Input: part model. Units: mm. Frame: model coordinates. A direction names the side the tool comes from. Give positions to 0.01 mm unless a question says otherwise; leave off trailing zeros. Write each loop counter-clockwise with the first axis right and the second up, starting at its lowest first coordinate (ties: lowest second). Pieces come first, ordered by that corner, then holes.
```python
from build123d import *

# Parameters (mm, degrees)
F1_DEPTH = 101
F2_W     = 28
F2_H     = 1
F3_DEPTH = 2


with BuildPart() as f1:
    # F0 (on Front) → F1 (new body)
    with BuildSketch(Plane.XZ):
        Polygon((19.7989898732, 1.4142135624), (0, 21.2132034356), (-0.4420594911, 18.826835802), (16.3847763109, 2), (-30.2015638745, 2), (-20.19282931, 38.5776056209), (-15.051559592, 33.4363359028), (-14.1421356237, 35.3553390593), (-21.2132034356, 42.4264068712), (-32.8223461799, 0), (-9.7140957444, 0), (21.2132034356, 0), align=None)
        Polygon((21.0717820794, 2.6870057685), (19.7989898732, 1.4142135624), (21.2132034356, 0), (23.9002092041, 2.6870057685), (21.0717820794, 5.5154328933), (19.657568517, 4.1012193309), align=None)
    extrude(amount=F1_DEPTH)

    # F2 (on face) → F3 (join)
    with BuildSketch(Plane(origin=(10.6066017178, 0, 10.6066017178), x_dir=(0.7071067812, 0, -0.7071067812), z_dir=(0.7071067812, 0, 0.7071067812))):
        with Locations((-1, -100.5)):
            Rectangle(F2_W, F2_H)
        with Locations((-1, -90.5)):
            Rectangle(F2_W, F2_H)
        with Locations((-1, -80.5)):
            Rectangle(F2_W, F2_H)
        with Locations((-1, -70.5)):
            Rectangle(F2_W, F2_H)
        with Locations((-1, -60.5)):
            Rectangle(F2_W, F2_H)
        with Locations((-1, -50.5)):
            Rectangle(F2_W, F2_H)
        with Locations((-1, -40.5)):
            Rectangle(F2_W, F2_H)
        with Locations((-1, -30.5)):
            Rectangle(F2_W, F2_H)
        with Locations((-1, -20.5)):
            Rectangle(F2_W, F2_H)
        with Locations((-1, -0.5)):
            Rectangle(F2_W, F2_H)
        with Locations((-1, -10.5)):
            Rectangle(F2_W, F2_H)
    extrude(amount=F3_DEPTH)


solid = f1.part
```
Q1. Section B-B, the plane x = -7. Return the cut outline in (y, z).
Q2. Section A-A, the plane y = -16.5. Return the cut outline in (x, z).
Q3. Section C-C, the plane z = 29.5. Return the cut outline in (x, y).
Q4. Pin query (flat end, axial travel): pin 1 (6 mm diameter, centred on y = -42.5, z = 26, fed in from +X); pin 2 (5 mm diameter, centred on y = -25, z = 31, fed in from +X); pin 3 (17 mm diameter, centred on x = 12.5, z = 11, fed in from +Y); pin 4 (6 mm diameter, centred on y = -36.5, z = 7, fed in from -X). Return the tip coordinate at first contact, or that it passes through.
Q5. Access query for faces 3 (the flat face through (-17.628, -49.793, 38.841)), 4 (the flat face through (-17.658, -49.793, 36.043)). Directions: +Z, -Z, +X, -X, +Y, -Y. A direction counts if a zero-diameter tool reaches every point of the face in a straight line with its end or side. Return the directions, or none.
Q6. Material intervals for line 1 along X through (y, z) = (-76, 3.5); line 2 along Z through (x, y) = (6, -39); line 3 along X through (y, z) = (-23.5, 4.5), sorted ascending.
Q7. Mould query, pull axis Y, two halves, no side actions, for faces 1 (the flat face through (10, -1, 12)), 2 (the flat face through (22.51, -49.79, 4.08)). Classes: +Y half, -Y half, draft (parallel to the pull), parting line (faces both ways), or undercut.
Solutions:
1. outline: (-101, 0) - (0, 0) - (0, 2) - (-101, 2) - close
2. outline: (-32.82, 0) - (21.21, 0) - (23.9, 2.69) - (21.07, 5.52) - (19.66, 4.1) - (21.07, 2.69) - (19.8, 1.41) - (0, 21.21) - (-0.44, 18.83) - (16.38, 2) - (-30.2, 2) - (-20.19, 38.58) - (-15.05, 33.44) - (-14.14, 35.36) - (-21.21, 42.43) - close
3. outline: (-24.75, -101) - (-22.68, -101) - (-22.68, 0) - (-24.75, 0) - close
4. pin 1: stops at x = -22.81
4. pin 2: stops at x = -15.02
4. pin 3: stops at y = 0
4. pin 4: stops at x = -31.73
5. face 3: +Z, +X, +Y, -Y
5. face 4: +Y, -Y
6. line 1: x = -31.86 to -29.79, 14.88 to 17.71, 20.26 to 23.09
6. line 2: z = 0 to 2, 12.38 to 15.21
6. line 3: x = -31.59 to -29.52, 13.88 to 16.71, 20.06 to 22.09
7. face 1: undercut
7. face 2: draft
